Design review of the part built by this model. Coordinates are the model's own, in mm. A direction names the side the tool comes from. Coordinates: 2 decimals unless noted, no trailing zeros. Order: outer loops, then holes, each group sorted by start corner. A loop starts at its lowest first (then second) coordinate and runs counter-clockwise, first axis right, second up. Notation, with made-up numbers: (79.5, 4) - (124.5, 4) arc R25 ccw to (124.5, 16) - close; hole circle Ø1 at (-15, 26.5). An arc over 180 degrees is marked (long way). Write each question's results on one line, items separated by ' | '. Start each with the question number.
```python
from build123d import *

# Parameters (mm, degrees)
SKETCH1_R           = 3.683
SKETCH1_W           = 26.416
SKETCH1_H           = 26.416
BOSS_EXTRUDE1_DEPTH = 25.4
SKETCH2_R           = 3.683
CUT_EXTRUDE1_DEPTH  = 39.1


with BuildPart() as part:
    # Sketch1 → Boss-Extrude1 (new body)
    with BuildSketch(Plane(origin=(0, 0, 0), x_dir=(1, 0, 0), z_dir=(0, 1, 0))):
        with BuildLine():
            Line((-50.8, 19.05), (50.8, 19.05))
            ThreePointArc((50.8, 19.05), (69.85, 0), (50.8, -19.05))
            Line((50.8, -19.05), (-50.8, -19.05))
            ThreePointArc((-50.8, -19.05), (-69.85, 0), (-50.8, 19.05))
        make_face()
        with Locations((-50.8, 0)):
            Circle(SKETCH1_R, mode=Mode.SUBTRACT)
        with Locations((50.8, 0)):
            Circle(SKETCH1_R, mode=Mode.SUBTRACT)
        Rectangle(SKETCH1_W, SKETCH1_H, mode=Mode.SUBTRACT)
    extrude(amount=BOSS_EXTRUDE1_DEPTH)

    # Sketch2 → Cut-Extrude1 (cut, through all)
    with BuildSketch(Plane.XY.offset(19.05)):
        with Locations((0, 12.7)):
            Circle(SKETCH2_R)
    extrude(amount=-CUT_EXTRUDE1_DEPTH, mode=Mode.SUBTRACT)


solid = part.part
```
(1) Mouldability with a two-part tool opening along X and no side actions: class faces 1 (the face through (-69.845, 12.522, 0.419)), 2 (the face through (-0.798, 9.105, 16.17)), 3 (the face through (-1, 18, -19.05)), 4 (the face through (69.845, 12.522, -0.419)) as +X half, -X half, draft (parallel to the pull), parting line (faces both ways), or undercut.
(2) Take a section at C-C (z = 0). State the section outline as (x, y) points, plus the area to 3 significant figures.
(3) To check wall thickness, follow line 1 along X through (y, z) = (8.75, 0); line 2 along Y through (x, z) = (0, 17); line 3 along Z through (x, y) = (50.8, 6.75). State the ranges of each line that lie inside material, in increasing order. Write a range as [from, to].
(4) Take a section at B-B (x = 0). State the section outline as (y, z) points.
(5) Take a section at A-A (y = 12.7). State the section outline as (x, z) points.
(6) Tool access review of faces 5 (the face through (-15, 25.4, 0)), 6 (the face through (13.208, 13, 0)): name each direction out of +Z, -Z, +X, -X, +Y, -Y from which nothing blocks a thin tool from reaching the whole face with its end or side.
(7) Clearance check with flat-ended pins moving along their axes: pin 1 (1 mm diameter, centred on x = -54, y = 4.5, fed in from -Z); pin 2 (2 mm diameter, centred on y = 18, z = -1.5, fed in from -X); pin 3 (1 mm diameter, centred on y = 16.5, z = -8, fed in from +X). State where each tip first meets the part, or that it passes through.
(8) Take a section at D-D (y = 6.75). State the section outline as (x, z) points, plus the area to 3 significant figures.
Worked out:
1) face 1: -X half | face 2: undercut | face 3: draft | face 4: +X half
2) outline: (-69.85, 0) - (-54.48, 0) - (-54.48, 25.4) - (-69.85, 25.4) - close; (-47.12, 0) - (-13.21, 0) - (-13.21, 25.4) - (-47.12, 25.4) - close; (13.21, 0) - (47.12, 0) - (47.12, 25.4) - (13.21, 25.4) - close; (54.48, 0) - (69.85, 0) - (69.85, 25.4) - (54.48, 25.4) - close | area: 2,500 mm^2
3) line 1: [-69.85, -54.48], [-47.12, -13.21], [13.21, 47.12], [54.48, 69.85] | line 2: [0, 9.02], [16.38, 25.4] | line 3: [-19.05, -3.68], [3.68, 19.05]
4) outline: (0, -19.05) - (9.02, -19.05) - (9.02, -13.21) - (0, -13.21) - close; (0, 13.21) - (9.02, 13.21) - (9.02, 19.05) - (0, 19.05) - close; (16.38, -19.05) - (25.4, -19.05) - (25.4, -13.21) - (16.38, -13.21) - close; (16.38, 13.21) - (25.4, 13.21) - (25.4, 19.05) - (16.38, 19.05) - close
5) outline: (-50.8, -19.05) - (-3.68, -19.05) - (-3.68, -13.21) - (-13.21, -13.21) - (-13.21, 13.21) - (-3.68, 13.21) - (-3.68, 19.05) - (-50.8, 19.05) arc R19.05 ccw to start; (3.68, -19.05) - (50.8, -19.05) arc R19.05 ccw to (50.8, 19.05) - (3.68, 19.05) - (3.68, 13.21) - (13.21, 13.21) - (13.21, -13.21) - (3.68, -13.21) - close; hole circle Ø7.37 at (-50.8, 0); hole circle Ø7.37 at (50.8, 0)
6) face 5: +Z, -Z, +X, -X, +Y | face 6: +Y, -Y
7) pin 1: z = -18.86 | pin 2: x = -69.84 | pin 3: x = 68.31
8) outline: (-50.8, -19.05) - (50.8, -19.05) arc R19.05 ccw to (50.8, 19.05) - (-50.8, 19.05) arc R19.05 ccw to start; hole circle Ø7.37 at (-50.8, 0); hole (-13.21, -13.21) - (13.21, -13.21) - (13.21, 13.21) - (-13.21, 13.21) - close; hole circle Ø7.37 at (50.8, 0) | area: 4,230 mm^2
